Part model, mm, in its own coordinate system. Face numbers are marked on the shaded views. A direction names the side the tool comes from. Give positions to 0.01 mm unless a question says otherwise; leave off trailing zeros. Order: outer loops, then holes, each group sorted by start corner. A loop starts at its lowest first (then second) coordinate and runs counter-clockwise, first axis right, second up. Notation, with made-up numbers: (-10.5, -34.5) - (9.5, -34.5) arc R19 cw to (9.5, -6.5) - close; hole circle Ø2 at (34.25, 80.5). An arc over 180 degrees is marked (long way). Use a Markdown table: item, result. Add a question column.
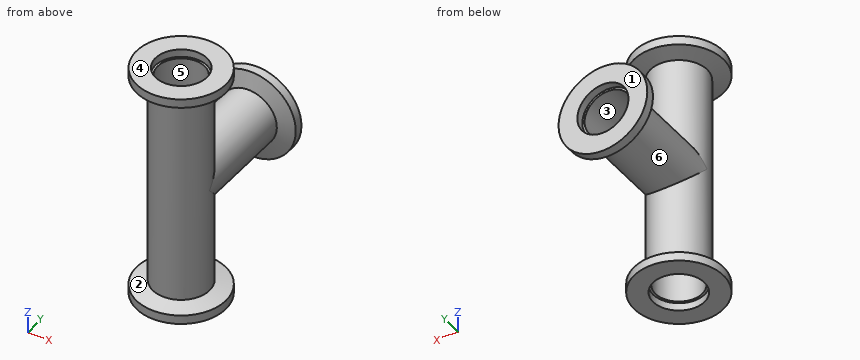
from build123d import *

# Parameters (mm, degrees)
CUT_EXTRUDE1_DEPTH      = 51.803373325
CUT_EXTRUDE1_DEPTH_BACK = 51.803373325
SKETCH4_R               = 7.874
CUT_EXTRUDE2_START      = -12.5095
SKETCH5_R               = 7.874
CUT_EXTRUDE2_DEPTH      = 64.312873325


with BuildPart() as part:
    # Sketch2 → Revolve1 (revolve)
    with BuildSketch(Plane(origin=(0, 0, 0), x_dir=(0, 0, -1), z_dir=(1, 0, 0)), mode=Mode.PRIVATE) as revolve1_sk:
        Polygon((-40.005, 2.4765), (-37.0078, 2.4765), (-35.54452946, -2.9845), (35.54452946, -2.9845), (37.0078, 2.4765), (40.005, 2.4765), (40.005, -3.8735), (37.3888, -3.8735), (37.3888, -12.5095), (-37.3888, -12.5095), (-37.3888, -3.8735), (-40.005, -3.8735), align=None)
    revolve(revolve1_sk.sketch.rotate(Axis((0, -12.5095, 40.005), (0, 0, -1)), 90), axis=Axis((0, -12.5095, 40.005), (0, 0, -1)))

    # Sketch3 → Revolve2 (revolve)
    with BuildSketch(Plane(origin=(0, 0, 0), x_dir=(0, 0, -1), z_dir=(1, 0, 0)), mode=Mode.PRIVATE) as revolve2_sk:
        Polygon((-14.986, 27.4955), (-14.986, 24.4983), (-9.525, 23.03502946), (-9.525, -12.5095), (0, -12.5095), (0, 24.8793), (-8.636, 24.8793), (-8.636, 27.4955), align=None)
    revolve(revolve2_sk.sketch.rotate(Axis((0, -12.5095, 0), (0, 1, 0)), 180), axis=Axis((0, -12.5095, 0), (0, 1, 0)))

    # Sketch4 → Cut-Extrude1 (cut, two sides: drawn at the far end of the back side and taken through both)
    with BuildSketch(Plane.XY.offset(-CUT_EXTRUDE1_DEPTH_BACK)):
        with Locations((0, -12.5095)):
            Circle(SKETCH4_R)
    extrude(amount=CUT_EXTRUDE1_DEPTH + CUT_EXTRUDE1_DEPTH_BACK, mode=Mode.SUBTRACT)

    # Sketch5 → Cut-Extrude2 (cut, through all)
    with BuildSketch(Plane(origin=(0, 0, 0), x_dir=(1, 0, 0), z_dir=(0, 1, 0)).offset(CUT_EXTRUDE2_START)):
        with Locations(Location((0, 0, 0), (0, 0, 90))):
            Circle(SKETCH5_R)
    extrude(amount=CUT_EXTRUDE2_DEPTH, mode=Mode.SUBTRACT)


solid = part.part
1. Cut at C-C (x = 0). State how many separate pieces and enclosed holes the cut face has, plus the area to 3 significant figures.
2. Tool access for the marked faces 1, 2 and 3: list every direction of +Z, -Z, +X, -X, +Y, -Y with a clear straight run to the whole face (end or side of a thin tool).
3. Mould opens along Z. For the marked faces 4, 5 and 6 say: released by +Z, released by -Z, zero draft, split by the parting line, or undercut.
4. Cut at B-B (y = 15). Write the cut outline in (x, z) (3 decimals), plus the area to 3 significant figures.
5. Pin check, flat tips, straight feed: P1, Ø3, axis at x = -8, z = -18.5, coming from the -Y side; P2, Ø3, axis at x = -6.5, z = -22, coming from the +Y side; P3, Ø14, axis at x = 0, y = -12.51, coming from the -Z side; P4, Ø9.5, axis at x = 0, z = 0, coming from the +Y side. Stop position of each tip, or through.
6. Drill centre lines: probe 1 along X at (y, z) = (5, 0) (3 decimals); probe 2 along Z at (x, y) = (-1, -1) (3 decimals); probe 3 along Y at (x, z) = (1.5, 12). Where is each one in solid material? Low to high. Write a range as [from, to].
Responses:
| question | item | result |
|---|---|---|
| 1 | separate pieces | 3 |
| 1 | enclosed holes | 0 |
| 1 | area | 449 mm² |
| 2 | face 1 | +Z, -Z, +X, -X, +Y |
| 2 | face 2 | none |
| 2 | face 3 | +Y |
| 3 | face 4 | released by +Z |
| 3 | face 5 | zero draft |
| 3 | face 6 | undercut |
| 4 | outline | circle Ø19.05 at (0, 0); hole circle Ø15.748 at (0, 0) |
| 4 | area | 90.2 mm² |
| 5 | P1 | stops at y = -19.47 |
| 5 | P2 | stops at y = -4.4 |
| 5 | P3 | passes through |
| 5 | P4 | stops at y = -18.79 |
| 6 | probe 1 | x = [-9.525, -7.874], [7.874, 9.525] |
| 6 | probe 2 | z = [-40.005, -36.088], [-9.472, -7.81], [7.81, 9.472], [36.088, 40.005] |
| 6 | probe 3 | y = [-21.92, -20.24], [-4.78, -3.1], [23.72, 27.5] |
